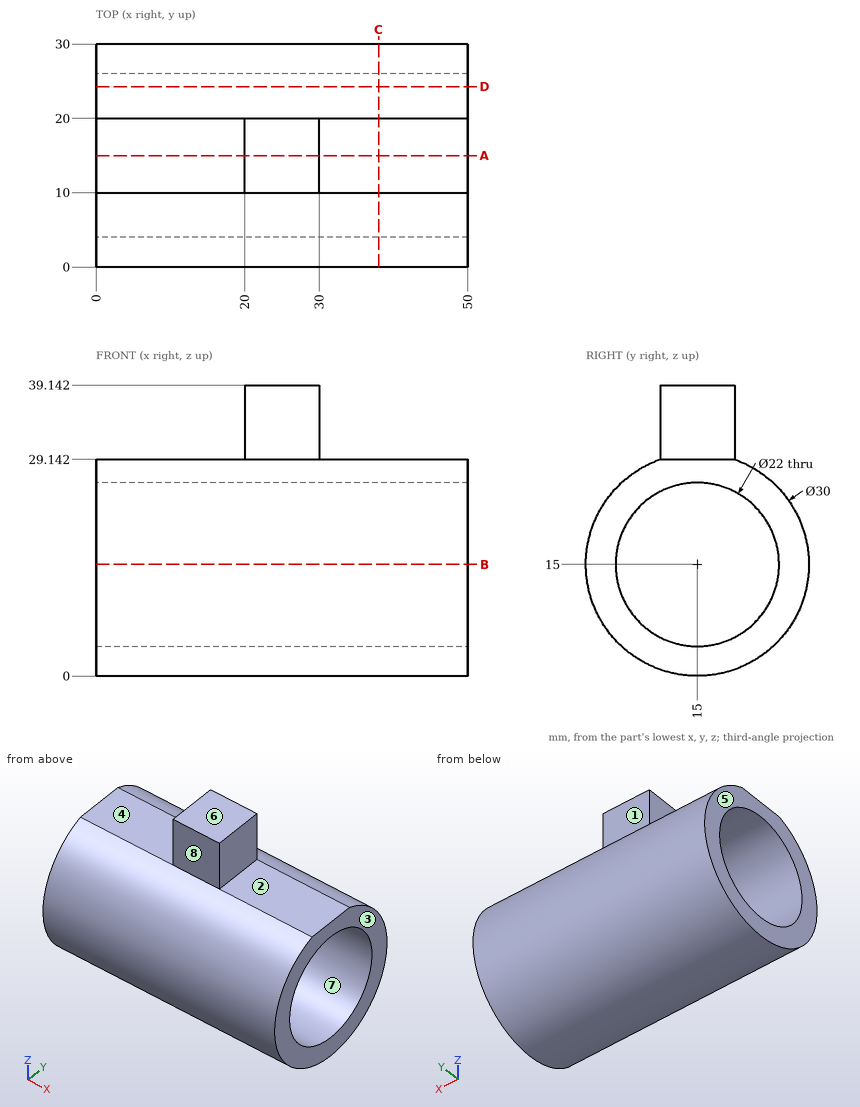
The drawing under review shows one solid part. Ordinate dimensions are in mm from its lowest x, y, z. A direction names the side the tool comes from. Round coordinates to 2 decimals unless told otherwise and drop trailing zeros. Loops run counter-clockwise (first coordinate to the right, second up) from the corner with the lowest first, then second, coordinate; pieces in that order, holes last. Notation, with made-up numbers: (-22.75, 56.5) - (26.25, 56.5) arc R25 ccw to (26.25, 95.5) - close; hole circle Ø3 at (12, 56). An arc over 180 degrees is marked (long way). One line per question, with ' | ' between items.
Q1. For line 1 along Y through (x, z) = (35.5, 15); line 2 along X through (y, z) = (16, 35); line 3 along Y through (x, z) = (21, 13), list the stretches that pass through material, from the lowest coordinate up. Write a range as [from, to].
Taken from the geometry:
line 1: y = [0, 4], [26, 30] | line 2: x = [20, 30] | line 3: y = [0.13, 4.18], [25.82, 29.87]
Q2. Take a section at D-D (y = 24.25). Give the boundary of the cut face in (x, z).
Taken from the geometry:
outline: (0, 3.19) - (50, 3.19) - (50, 9.05) - (0, 9.05) - close; (0, 20.95) - (50, 20.95) - (50, 26.81) - (0, 26.81) - close
Q3. Take a section at A-A (y = 15). Give the boundary of the cut face in (x, z).
Taken from the geometry:
outline: (0, 0) - (50, 0) - (50, 4) - (0, 4) - close; (0, 26) - (50, 26) - (50, 29.14) - (30, 29.14) - (30, 39.14) - (20, 39.14) - (20, 29.14) - (0, 29.14) - close
Q4. Take a section at C-C (x = 38). Give the boundary of the cut face in (y, z), and give its area (3 significant figures).
Taken from the geometry:
outline: (10, 29.14) arc R15 ccw (long way) to (20, 29.14) - close; hole circle Ø22 at (15, 15) | area: 321 mm²
Q5. For pin 1 (8 mm diameter, centred on x = 6, y = 13.5, fed in from +Z); pin 2 (8 mm diameter, centred on y = 17, z = 33.5, fed in from -X); pin 3 (4 mm diameter, centred on x = 18.5, z = 19.5, fed in from -Y), all flat-tipped, find the tip position at first contact; note any pin that passes through.
Taken from the geometry:
pin 1: stops at z = 29.14 | pin 2: stops at x = 20 | pin 3: stops at y = 0.21
Q6. The part is to be moulded in two halves that separate along Y. For the marked faces 6, 7 and 8, say which applies: released by +Y, released by -Y, zero draft, split by the parting line, or undercut.
Taken from the geometry:
face 6: zero draft | face 7: undercut | face 8: released by -Y
Q7. Tool access review of the marked faces 1, 2, 3, 4 and 5: name each direction out of +Z, -Z, +X, -X, +Y, -Y from which nothing blocks a thin tool from reaching the whole face with its end or side.
Taken from the geometry:
face 1: +Z, +X, -X, +Y | face 2: +Z, +X, +Y, -Y | face 3: +Z, -Z, +X, +Y, -Y | face 4: +Z, -X, +Y, -Y | face 5: +Z, -Z, -X, +Y, -Y
Q8. Take a section at B-B (z = 15). Give the boundary of the cut face in (x, y), and give its area (3 significant figures).
Taken from the geometry:
outline: (0, 0) - (50, 0) - (50, 4) - (0, 4) - close; (0, 26) - (50, 26) - (50, 30) - (0, 30) - close | area: 400 mm²
